```python
from build123d import *

# Parameters (mm, degrees)
SKETCH1_R             = 1.55
BOSS_EXTRUDE1_DEPTH   = 70
BOSS_EXTRUDE1_2_DEPTH = 70
BOSS_EXTRUDE1_3_DEPTH = 70
BOSS_EXTRUDE1_4_DEPTH = 70
SKETCH2_W             = 164.9
SKETCH2_H             = 213
BOSS_EXTRUDE2_DEPTH   = 2
SKETCH3_R             = 1.55
CUT_EXTRUDE1_DEPTH    = 10


with BuildPart() as part:
    # Sketch1 → Boss-Extrude1 (new body)
    with BuildSketch(Plane(origin=(0, 0, 0), x_dir=(1, 0, 0), z_dir=(0, 1, 0))):
        with Locations(Location((-80.9, 29.78, 0), (0, 0, 270))):
            Circle(SKETCH1_R)
    extrude(amount=BOSS_EXTRUDE1_DEPTH)



with BuildPart() as body_2:
    # Sketch1 → Boss-Extrude1 2 (new body)
    with BuildSketch(Plane(origin=(0, 0, 0), x_dir=(1, 0, 0), z_dir=(0, 1, 0))):
        with Locations(Location((-80.9, -29.78, 0), (0, 0, 270))):
            Circle(SKETCH1_R)
    extrude(amount=BOSS_EXTRUDE1_2_DEPTH)


with BuildPart() as body_3:
    # Sketch1 → Boss-Extrude1 3 (new body)
    with BuildSketch(Plane(origin=(0, 0, 0), x_dir=(1, 0, 0), z_dir=(0, 1, 0))):
        with Locations(Location((80.9, 29.78, 0), (0, 0, 270))):
            Circle(SKETCH1_R)
    extrude(amount=BOSS_EXTRUDE1_3_DEPTH)


with BuildPart() as body_4:
    # Sketch1 → Boss-Extrude1 4 (new body)
    with BuildSketch(Plane(origin=(0, 0, 0), x_dir=(1, 0, 0), z_dir=(0, 1, 0))):
        with Locations(Location((80.9, -29.78, 0), (0, 0, 270))):
            Circle(SKETCH1_R)
    extrude(amount=BOSS_EXTRUDE1_4_DEPTH)


with BuildPart() as part_1:
    add(part.part)

    add(body_2.part)  # Boss-Extrude2 merges body 2

    add(body_3.part)  # Boss-Extrude2 merges body 3

    add(body_4.part)  # Boss-Extrude2 merges body 4
    # Sketch2 → Boss-Extrude2 (add)
    with BuildSketch(Plane(origin=(0, 0, 0), x_dir=(1, 0, 0), z_dir=(0, 1, 0))):
        Rectangle(SKETCH2_W, SKETCH2_H)
    extrude(amount=BOSS_EXTRUDE2_DEPTH)

    # Sketch3 → Cut-Extrude1 (cut)
    with BuildSketch(Plane(origin=(0, 2, 0), x_dir=(1, 0, 0), z_dir=(0, 1, 0))):
        with Locations(Location((-52.45, 76.5, 0), (0, 0, 270))):
            Circle(SKETCH3_R)
        with Locations(Location((52.45, 76.5, 0), (0, 0, 270))):
            Circle(SKETCH3_R)
        with Locations(Location((52.45, -76.5, 0), (0, 0, 270))):
            Circle(SKETCH3_R)
        with Locations(Location((-52.45, -76.5, 0), (0, 0, 270))):
            Circle(SKETCH3_R)
    extrude(amount=-CUT_EXTRUDE1_DEPTH, mode=Mode.SUBTRACT)


solid = part_1.part
```
The listing builds one solid part. Answer for the finished solid, in the listing's coordinates (mm). Give positions to 0.01 mm unless a question says otherwise; leave off trailing zeros. Order: outer loops, then holes, each group sorted by start corner. A loop starts at its lowest first (then second) coordinate and runs counter-clockwise, first axis right, second up. Notation, with made-up numbers: (-3.5, 4) -> (21.5, 4) arc R30 ccw to (21.5, 29) -> close; hole circle Ø5 at (41, 10.25). An arc over 180 degrees is marked (long way). Answer as CSV lines item,"result". Start each with the question number.
Q1. A cutting plane is placed at B-B (x = 67). Determine the outline of the cut face in (y, z).
Q2. Given pin 1 (1.9 mm diameter, centred on x = -52.45, z = 76.5, fed in from +Y); pin 2 (5 mm diameter, centred on x = -12.5, z = -20.5, fed in from +Y), each flat-ended and moving along its own axis, determine where each tip first touches the part or whether it passes through.
Q3. A cutting plane is placed at A-A (y = 64). Determine the outline of the cut face in (x, z).
Q4. A cutting plane is placed at C-C (z = -41.5). Determine the outline of the cut face in (x, y), then the cut area to 3 significant figures.
Q5. Find the intervals of material crossed by L1, parallel to X at y = 1.3, z = 76.5; L2, parallel to Y at x = 58, z = 74; L3, parallel to X at y = 1, z = -76, in increasing order.
Results found:
1,outline,"(0, -106.5) -> (2, -106.5) -> (2, 106.5) -> (0, 106.5) -> close"
2,pin 1,"through"
2,pin 2,"y = 2"
3,outline,"circle Ø3.1 at (-80.9, -29.78); circle Ø3.1 at (-80.9, 29.78); circle Ø3.1 at (80.9, -29.78); circle Ø3.1 at (80.9, 29.78)"
4,outline,"(-82.45, 0) -> (82.45, 0) -> (82.45, 2) -> (-82.45, 2) -> close"
4,area,"330 mm2"
5,L1,"-82.45 to -54, -50.9 to 50.9, 54 to 82.45"
5,L2,"0 to 2"
5,L3,"-82.45 to -53.92, -50.98 to 50.98, 53.92 to 82.45"
